Design review of the part built by this model. Coordinates are the model's own, in mm. A direction names the side the tool comes from. Give positions to 0.01 mm unless a question says otherwise; leave off trailing zeros. Loops run counter-clockwise (first coordinate to the right, second up) from the corner with the lowest first, then second, coordinate; pieces in that order, holes last. Notation, with made-up numbers: (21, 22) - (26, 22) arc R18 cw to (26, 50) - close; hole circle Ø9 at (-2, 68). An arc over 180 degrees is marked (long way). Write each question's results on one line, items separated by ' | '.
from build123d import *

# Parameters (mm, degrees)
SKETCH1_W           = 100
SKETCH1_H           = 75
BOSS_EXTRUDE1_DEPTH = 5
SKETCH2_W           = 75
SKETCH2_H           = 100
SKETCH2_W_2         = 65
SKETCH2_H_2         = 90
BOSS_EXTRUDE2_DEPTH = 3
SKETCH3_W           = 15
SKETCH3_H           = 25
CUT_EXTRUDE1_DEPTH  = 63.69968102
FILLET1_R           = 5
FILLET2_R           = 1


with BuildPart() as part:
    # Sketch1 → Boss-Extrude1 (new body)
    with BuildSketch(Plane(origin=(0, 0, 0), x_dir=(0, 1, 0), z_dir=(0, 0, 1))):
        Rectangle(SKETCH1_W, SKETCH1_H)
    extrude(amount=BOSS_EXTRUDE1_DEPTH)

    # Sketch2 → Boss-Extrude2 (add)
    with BuildSketch(Plane.XY.offset(5)):
        Rectangle(SKETCH2_W, SKETCH2_H)
        Rectangle(SKETCH2_W_2, SKETCH2_H_2, mode=Mode.SUBTRACT)
    extrude(amount=BOSS_EXTRUDE2_DEPTH)

    # Sketch3 → Cut-Extrude1 (cut, through all)
    with BuildSketch(Plane.XY.offset(5)):
        with Locations((-25, 32.5)):
            Rectangle(SKETCH3_W, SKETCH3_H)
        with BuildLine():
            Line((-2.15, 2.15), (2.15, 2.15))
            ThreePointArc((2.15, 2.15), (4.3, 0), (2.15, -2.15))
            Line((2.15, -2.15), (-2.15, -2.15))
            ThreePointArc((-2.15, -2.15), (-4.3, 0), (-2.15, 2.15))
        make_face()
    extrude(amount=-CUT_EXTRUDE1_DEPTH, mode=Mode.SUBTRACT)

    # Fillet1
    fillet1_edges = [part.edges().sort_by_distance(p)[0] for p in [
        (37.5, 50, 4),
        (37.5, -50, 4),
        (-37.5, -50, 4),
        (-37.5, 50, 4),
    ]]
    fillet(fillet1_edges, radius=FILLET1_R)

    # Fillet2
    fillet2_edges = [part.edges().sort_by_distance(p)[0] for p in [
        (32.5, 0, 8),
        (0, 45, 8),
        (-32.5, 0, 8),
        (0, -45, 8),
        (-25, 20, 5),
        (-17.5, 32.5, 5),
    ]]
    fillet(fillet2_edges, radius=FILLET2_R)


solid = part.part
(1) Take a section at C-C on x = -30.5. Give the boundary of the cut face in (y, z), plus the area to 3 significant figures.
Answers below:
outline: (-50, 0) - (20, 0) - (20, 4) arc R1 ccw to (19, 5) - (-45, 5) - (-45, 7) arc R1 ccw to (-46, 8) - (-50, 8) - close; (45, 0) - (50, 0) - (50, 8) - (46, 8) arc R1 ccw to (45, 7) - close | area: 404 mm2
(2) Take a section at A-A on y = 26. Give the boundary of the cut face in (x, z), plus the area to 3 significant figures.
Answers below:
outline: (-37.5, 0) - (-32.5, 0) - (-32.5, 7) arc R1 ccw to (-33.5, 8) - (-37.5, 8) - close; (-17.5, 0) - (37.5, 0) - (37.5, 8) - (33.5, 8) arc R1 ccw to (32.5, 7) - (32.5, 5) - (-16.5, 5) arc R1 ccw to (-17.5, 4) - close | area: 329 mm2
(3) Wall thickness on line 1 along Y through (x, z) = (31, 6); line 2 along X through (y, z) = (19, 6.5); line 3 along X through (y, z) = (44, 3.5): over which ranges is each line inside the solid? List them lowest first. Write a range as from..to.
Answers below:
line 1: -50..-45, 45..50 | line 2: -37.5..-32.5, 32.5..37.5 | line 3: -37.5..-32.5, -17.5..37.5
(4) Tool access review of faces 5 (the flat face through (32.5, -1, 6)), 6 (the flat face through (8, -1, 0)), 7 (the cylindrical face through (-4.3, 0, 2.5)): name each direction out of +Z, -Z, +X, -X, +Y, -Y from which nothing blocks a thin tool from reaching the whole face with its end or side.
Answers below:
face 5: +Z | face 6: -Z, +X, -X, +Y, -Y | face 7: +Z, -Z
(5) Take a section at D-D on y = -38. Give the boundary of the cut face in (x, z), plus the area to 3 significant figures.
Answers below:
outline: (-37.5, 0) - (37.5, 0) - (37.5, 8) - (33.5, 8) arc R1 ccw to (32.5, 7) - (32.5, 5) - (-32.5, 5) - (-32.5, 7) arc R1 ccw to (-33.5, 8) - (-37.5, 8) - close | area: 405 mm2
(6) Draft analysis for pull direction X (two halves, no side actions). For faces 1 (the cylindrical face through (-36.07, 48.5, 3.94)), 2 (the flat face through (37.5, -1, 4)), 3 (the flat face through (-25, 20, 2)), 4 (the flat face through (0, -50, 4)), state which applies: pulls with the +X half, pulls with the -X half, needs draft (parallel to the pull), parting line crosses it, or undercut.
Answers below:
face 1: pulls with the -X half | face 2: pulls with the +X half | face 3: undercut | face 4: needs draft
(7) Take a section at B-B on z = 1.25. Give the boundary of the cut face in (x, y).
Answers below:
outline: (-37.5, -45) arc R5 ccw to (-32.5, -50) - (32.5, -50) arc R5 ccw to (37.5, -45) - (37.5, 45) arc R5 ccw to (32.5, 50) - (-32.5, 50) arc R5 ccw to (-37.5, 45) - close; hole (-32.5, 20) - (-17.5, 20) - (-17.5, 45) - (-32.5, 45) - close; hole (-2.15, -2.15) - (2.15, -2.15) arc R2.15 ccw to (2.15, 2.15) - (-2.15, 2.15) arc R2.15 ccw to start
(8) Insertion check: P1, Ø19.5, axis at x = -5.5, y = 4, coming from the +Z side; P2, Ø10, axis at x = -14.5, y = -29.5, coming from the -Z side. Each pin has a flat end and moves straight along its axis. Give the tip position at first contact, or say it passes through.
Answers below:
P1: z = 5 | P2: z = 0
